from build123d import *

# Parameters (mm, degrees)
EXTRUDE_1_DEPTH              = 14.5
HOLE_START                   = -15
HOLE_WIZARD_M2_1_OUTLINE_R   = 1.9
HOLE_WIZARD_M2_1_DEPTH       = 1
HOLE_START_2                 = -14
HOLE_WIZARD_M2_1_2_OUTLINE_R = 1.05
HOLE_WIZARD_M2_1_2_DEPTH     = 1
SKETCH_5_R                   = 8
EXTRUDE_2_DEPTH              = 2.5
SKETCH_10_W                  = 3
SKETCH_10_H                  = 10
CUT_EXTRUDE_4_DEPTH          = 37.087567111
SKETCH_9_W                   = 13
SKETCH_9_H                   = 5
CUT_EXTRUDE_3_DEPTH          = 37.087567111
FILLET_1_R                   = 4
CUT_EXTRUDE_START            = -2.5
CUT_EXTRUDE_5_OUTLINE_R      = 6.25
CUT_EXTRUDE_5_DEPTH          = 2.5
HOLE_WIZARD_M2_2_D           = 2.1
HOLE_WIZARD_M2_2_CBORE_D     = 3.8
HOLE_WIZARD_M2_2_CBORE_DEPTH = 1
FILLET_4_R                   = 2.5
FILLET_5_R                   = 1
SKETCH_14_W                  = 9
SKETCH_14_H                  = 26
EXTRUDE_4_DEPTH              = 6.5
CUT_EXTRUDE_6_REACH          = 33.001
SKETCH_15_W                  = 20
SKETCH_15_H                  = 4
CUT_EXTRUDE_7_REACH          = 38.088
SKETCH_16_W                  = 5
SKETCH_16_H                  = 4
CUT_EXTRUDE_8_REACH          = 28.448
SKETCH_17_W                  = 5
SKETCH_17_H                  = 19
CUT_EXTRUDE_9_DEPTH          = 37.087567111
FILLET_6_R                   = 1


# Read off the part's stored shape, not the designer's step: M2 丸平ねじ用座ぐり穴1, ｶｯﾄ - 押し出し5
with BuildPart() as part:
    # ｽｹｯﾁ1 → ﾎﾞｽ - 押し出し1 (new, symmetric)
    with BuildSketch(Plane(origin=(0, 0, 0), x_dir=(0, 0, -1), z_dir=(1, 0, 0))):
        Polygon((-15, -7.75), (15, -7.75), (15, 7.75), (13, 7.75), (13, -5.25), (-13, -5.25), (-13, 7.75), (-15, 7.75), align=None)
    extrude(amount=EXTRUDE_1_DEPTH, both=True)

    # M2 丸平ねじ用座ぐり穴1 outline → M2 丸平ねじ用座ぐり穴1 (cut)
    with BuildSketch(Plane.XY.offset(HOLE_START)):
        with Locations((-10.5, 3.75)):
            Circle(HOLE_WIZARD_M2_1_OUTLINE_R)
        with Locations((10.5, 3.75)):
            Circle(HOLE_WIZARD_M2_1_OUTLINE_R)
    hole_wizard_m2_1 = extrude(amount=HOLE_WIZARD_M2_1_DEPTH, mode=Mode.SUBTRACT)

    # Hole Wizard M2 _1 2 outline → Hole Wizard M2 _1 2 (cut)
    with BuildSketch(Plane.XY.offset(HOLE_START_2)):
        with Locations((-10.5, 3.75)):
            Circle(HOLE_WIZARD_M2_1_2_OUTLINE_R)
        with Locations((10.5, 3.75)):
            Circle(HOLE_WIZARD_M2_1_2_OUTLINE_R)
    hole_wizard_m2_1_2 = extrude(amount=HOLE_WIZARD_M2_1_2_DEPTH, mode=Mode.SUBTRACT)

    # ｽｹｯﾁ5 → ﾎﾞｽ - 押し出し2 (add)
    with BuildSketch(Plane.XZ.offset(7.75)):
        with Locations((-10.5, 0)):
            Circle(SKETCH_5_R)
    extrude(amount=-EXTRUDE_2_DEPTH)

    # ｽｹｯﾁ10 → ｶｯﾄ - 押し出し4 (cut, through all)
    with BuildSketch(Plane(origin=(0, 0, -15), x_dir=(-1, 0, 0), z_dir=(0, 0, -1))):
        with Locations((-14.5, -5.25)):
            Rectangle(SKETCH_10_W, SKETCH_10_H)
    extrude(amount=-CUT_EXTRUDE_4_DEPTH, mode=Mode.SUBTRACT)

    # ｽｹｯﾁ9 → ｶｯﾄ - 押し出し3 (cut, through all)
    with BuildSketch(Plane(origin=(0, 0, -15), x_dir=(-1, 0, 0), z_dir=(0, 0, -1))):
        with Locations((10, -2.75)):
            Rectangle(SKETCH_9_W, SKETCH_9_H)
    extrude(amount=-CUT_EXTRUDE_3_DEPTH, mode=Mode.SUBTRACT)

    # ﾌｨﾚｯﾄ1
    fillet_1_edges = [part.edges().sort_by_distance(p)[0] for p in [
        (-14.5, 7.75, 14),
        (14.5, 7.75, 14),
        (14.5, 7.75, -14),
        (-14.5, 7.75, -14),
        (-14.5, -0.25, 14),
        (-14.5, -0.25, -14),
    ]]
    fillet(fillet_1_edges, radius=FILLET_1_R - 0.0001)  # a hair under: the kernel refuses the full size

    # ｶｯﾄ - 押し出し5 outline → ｶｯﾄ - 押し出し5 (cut)
    with BuildSketch(Plane.XZ.offset(7.75).offset(CUT_EXTRUDE_START)):
        with BuildLine():
            Line((-14.5, -15), (-3.5, -15))
            Line((-3.5, -15), (-3.5, -10.95445115))
            ThreePointArc((-3.5, -10.95445115), (-8.076137007, -12.772035397), (-13, -12.757350822))
            Line((-13, -12.757350822), (-13, -7.599342077))
            ThreePointArc((-13, -7.599342077), (-13.7672782, -7.302389552), (-14.5, -6.92820323))
            Line((-14.5, -6.92820323), (-14.5, -15))
        make_face()
        with BuildLine():
            Line((-14.5, 15), (-14.5, 6.92820323))
            ThreePointArc((-14.5, 6.92820323), (-13.7672782, 7.302389552), (-13, 7.599342077))
            Line((-13, 7.599342077), (-13, 12.757350822))
            ThreePointArc((-13, 12.757350822), (-8.076137007, 12.772035397), (-3.5, 10.95445115))
            Line((-3.5, 10.95445115), (-3.5, 15))
            Line((-3.5, 15), (-14.5, 15))
        make_face()
        with Locations((-10.5, 0)):
            Circle(CUT_EXTRUDE_5_OUTLINE_R)
    extrude(amount=CUT_EXTRUDE_5_DEPTH, mode=Mode.SUBTRACT)

    # M2 丸平ねじ用座ぐり穴2 (through all)
    with Locations(Plane(origin=(0, -5.25, 0), x_dir=(1, 0, 0), z_dir=(0, 1, 0))):
        with Locations((10.5, -10.5), (10.5, 10.5), (-10.5, 10.5), (-10.5, -10.5)):
            CounterBoreHole(HOLE_WIZARD_M2_2_D / 2, HOLE_WIZARD_M2_2_CBORE_D / 2, HOLE_WIZARD_M2_2_CBORE_DEPTH)

    # ﾌｨﾚｯﾄ4
    fillet_4_edges = [part.edges().sort_by_distance(p)[0] for p in [
        (-13, -6.5, -12.757350822),
        (-13, -6.5, 12.757350822),
    ]]
    fillet(fillet_4_edges, radius=FILLET_4_R - 0.0001)  # a hair under: the kernel refuses the full size

    # ﾌｨﾚｯﾄ5
    fillet_5_edges = [part.edges().sort_by_distance(p)[0] for p in [
        (-3.5, -6.5, -10.95445115),
        (-13, -6.5, -7.599342077),
        (-13, -6.5, 7.599342077),
        (-3.5, -6.5, 10.95445115),
    ]]
    fillet(fillet_5_edges, radius=FILLET_5_R)

    # ｽｹｯﾁ14 → ﾎﾞｽ - 押し出し4 (add)
    with BuildSketch(Plane(origin=(0, -5.25, 0), x_dir=(1, 0, 0), z_dir=(0, 1, 0))):
        with Locations((3, 0)):
            Rectangle(SKETCH_14_W, SKETCH_14_H)
    extrude(amount=EXTRUDE_4_DEPTH)

    # ｽｹｯﾁ15 → ｶｯﾄ - 押し出し6 (cut, up to next)
    with BuildSketch(Plane(origin=(7.5, 0, 0), x_dir=(0, 0, -1), z_dir=(1, 0, 0)), mode=Mode.PRIVATE) as cut_extrude_6_sk1:
        with Locations((0, -0.75)):
            Rectangle(SKETCH_15_W, SKETCH_15_H)
    cut_extrude_6_tool1 = extrude(cut_extrude_6_sk1.sketch, amount=-CUT_EXTRUDE_6_REACH, mode=Mode.PRIVATE) & part.part
    add(cut_extrude_6_tool1.solids().sort_by_distance((7.5, -0.75, 0))[0], mode=Mode.SUBTRACT)

    # ｽｹｯﾁ16 → ｶｯﾄ - 押し出し7 (cut, up to next)
    with BuildSketch(Plane(origin=(0, 0, -15), x_dir=(-1, 0, 0), z_dir=(0, 0, -1)), mode=Mode.PRIVATE) as cut_extrude_7_sk1:
        with Locations((-3, -5.75)):
            Rectangle(SKETCH_16_W, SKETCH_16_H)
    cut_extrude_7_tool1 = extrude(cut_extrude_7_sk1.sketch, amount=-CUT_EXTRUDE_7_REACH, mode=Mode.PRIVATE) & part.part
    add(cut_extrude_7_tool1.solids().sort_by_distance((3, -5.75, -15))[0], mode=Mode.SUBTRACT)

    # ｽｹｯﾁ17 → ｶｯﾄ - 押し出し8 (cut, up to next)
    with BuildSketch(Plane.XZ.offset(3.75), mode=Mode.PRIVATE) as cut_extrude_8_sk1:
        with Locations((3, 0)):
            Rectangle(SKETCH_17_W, SKETCH_17_H)
    cut_extrude_8_tool1 = extrude(cut_extrude_8_sk1.sketch, amount=-CUT_EXTRUDE_8_REACH, mode=Mode.PRIVATE) & part.part
    add(cut_extrude_8_tool1.solids().sort_by_distance((3, -3.75, 0))[0], mode=Mode.SUBTRACT)

    # ﾐﾗｰ1: M2 丸平ねじ用座ぐり穴1, Hole Wizard M2 _1 2 across plane
    add(hole_wizard_m2_1.mirror(Plane.XY), mode=Mode.SUBTRACT)
    add(hole_wizard_m2_1_2.mirror(Plane.XY), mode=Mode.SUBTRACT)

    # ｽｹｯﾁ18 → ｶｯﾄ - 押し出し9 (cut, through all)
    with BuildSketch(Plane(origin=(0, 0, -15), x_dir=(-1, 0, 0), z_dir=(0, 0, -1))):
        with BuildLine():
            Line((-14.5, 3.75), (-14.5, -0.25))
            Line((-14.5, -0.25), (-13, -0.25))
            Line((-13, -0.25), (-13, 0.627501001))
            ThreePointArc((-13, 0.627501001), (-14.105551275, 2.017949192), (-14.5, 3.75))
        make_face()
    extrude(amount=-CUT_EXTRUDE_9_DEPTH, mode=Mode.SUBTRACT)

    # ﾌｨﾚｯﾄ6
    fillet_6_edges = [part.edges().sort_by_distance(p)[0] for p in [
        (7.5, -2.75, 0),
        (-1.5, -2.75, 0),
        (-1.5, -7.75, -15),
        (-1.5, -7.75, 15),
        (13, 0.627501001, 14),
        (13, 0.627501001, -14),
        (9.25, -7.75, -15),
        (9.25, -7.75, 15),
        (-3.5, -0.25, 14),
        (-3.5, -0.25, -14),
    ]]
    fillet(fillet_6_edges, radius=FILLET_6_R)


solid = part.part
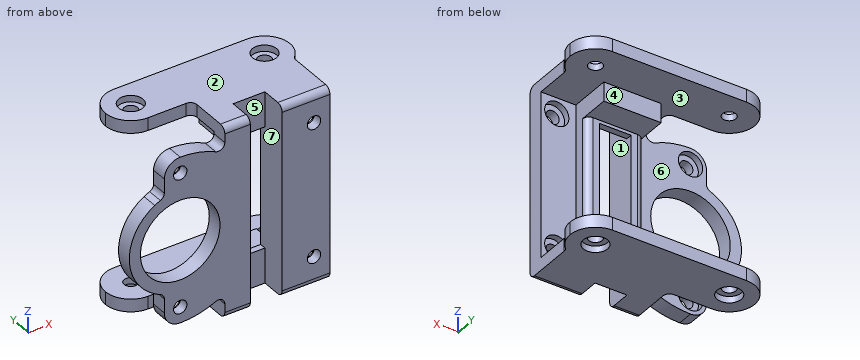
Here's how the part is built. I have some questions about the finished solid (model axes, mm). Face numbers are marked on the shaded views. A direction names the side the tool comes from. Coordinates: 2 decimals unless noted, no trailing zeros. Write each loop counter-clockwise with the first axis right and the second up, starting at its lowest first coordinate (ties: lowest second). Pieces come first, ordered by that corner, then holes. Notation, with made-up numbers: (80, 37) - (95, 37) arc R21 cw to (95, 68) - close; hole circle Ø4 at (-19, 53). An arc over 180 degrees is marked (long way). Use one line per item in the form item = value.
1) On a 3-axis mill with a long thin cutter (end or side, diameter ignored), from which of +Z, -Z, +X, -X, +Y, -Y can I reach the whole of each face in a straight line? I mean the marked faces 3, 4, 5, 6 and 7. Say none if no direction works.
Solved:
face_3 = +Y
face_4 = +X, -X, +Y
face_5 = +Z, -Z, -Y
face_6 = -X, +Y
face_7 = -Y
2) Thinking about a two-plate mould opening in X: for the marked faces 1 and 2, which applies, released by +X, released by -X, zero draft, split by the parting line, or undercut?
Solved:
face_1 = undercut
face_2 = zero draft
3) Suppose I cut it at D-D, the plane x = -12. Give the number of separate pieces and of enclosed holes in the cut face, plus the area to 3 significant figures.
Solved:
separate_pieces = 4
enclosed_holes = 0
area = 52.5 mm2
4) I'm going to push flat-ended pins straight in: P1, Ø1.8, axis at y = -6, z = 9.5, coming from the -X side; P2, Ø3.5, axis at x = -10.5, y = 3.75, coming from the -Z side; P3, Ø5, axis at y = -1.5, z = -3.5, coming from the -X side. Where does each tip first touch, or does it pass through?
Solved:
P1 = -13
P2 = -14
P3 = -1.5
5) Suppose I cut it at A-A, the plane y = -4.75. Write out the boundary of the cut face in (x, z), plus the area to 3 significant figures.
Solved:
outline = (-3.5, -15) - (0.5, -15) - (0.5, 15) - (-3.5, 15) - (-3.5, 13) - (-1.5, 13) - (-1.5, -13) - (-3.5, -13) - close; (5.5, -15) - (13, -15) - (13, -13) - (7.5, -13) - (7.5, 13) - (13, 13) - (13, 15) - (5.5, 15) - close
area = 150 mm2
6) Suppose I cut it at B-B, the plane z = 0. Write out the boundary of the cut face in (x, y), plus the area to 3 significant figures.
Solved:
outline = (-18.5, -7.75) - (-16.75, -7.75) - (-16.75, -5.25) - (-18.5, -5.25) - close; (-4.25, -7.75) - (0.5, -7.75) - (0.5, -2.75) - (-0.5, -2.75) arc R1 ccw to (-1.5, -3.75) - (-1.5, -5.25) - (-4.25, -5.25) - close; (5.5, -7.75) - (13, -7.75) - (13, -5.25) - (7.5, -5.25) - (7.5, -3.75) arc R1 ccw to (6.5, -2.75) - (5.5, -2.75) - close
area = 44.6 mm2
7) Suppose I cut it at C-C, the plane x = 1. Write out the boundary of the cut face in (y, z).
Solved:
outline = (-3.75, -15) - (7.75, -15) - (7.75, -13) - (1.25, -13) - (1.25, -10) - (-2.75, -10) - (-2.75, -9.5) - (-3.75, -9.5) - close; (-3.75, 9.5) - (-2.75, 9.5) - (-2.75, 10) - (1.25, 10) - (1.25, 13) - (7.75, 13) - (7.75, 15) - (-3.75, 15) - close
8) I need wall thicknesses on line 1 (X direction, y = -5.6, z = 10.5); line 2 (X direction, y = -6.8, z = 10.5); line 3 (Y direction, x = -10.5, z = 14.75). Which ranges of each line are inside material? Lowest first, please.
Solved:
line_1 = -13 to -12.4, -8.6 to 0.5, 5.5 to 8.6, 12.4 to 13
line_2 = -13 to -11.55, -9.45 to 0.5, 5.5 to 9.45, 11.55 to 13
line_3 = -0.25 to 1.85, 5.65 to 7.75
